Geometry: final body of the model. Coordinates: model frame, mm. A direction names the side the tool comes from. Coordinates: 2 decimals unless noted, no trailing zeros. Order: outer loops, then holes, each group sorted by start corner. A loop starts at its lowest first (then second) coordinate and runs counter-clockwise, first axis right, second up. Notation, with made-up numbers: (35, 67) -> (91, 67) arc R21 ccw to (91, 81) -> close; hole circle Ø2 at (-2, 12.25). An arc over 180 degrees is marked (long way). Use one line per item in the form item = value.
```python
from build123d import *

# Parameters (mm, degrees)
SKETCH1_R           = 1.475
SKETCH1_R_2         = 22.5
SKETCH1_R_3         = 11
SKETCH1_W           = 24.7
SKETCH1_H           = 4.85
BOSS_EXTRUDE1_DEPTH = 5


with BuildPart() as part:
    # Sketch1 → Boss-Extrude1 (new body)
    with BuildSketch(Plane.XY):
        with BuildLine():
            Line((-139.300035894, 89.802561211), (-24.748737342, -24.748737342))
            ThreePointArc((-24.748737342, -24.748737342), (24.748737342, -24.748737342), (24.748737342, 24.748737342))
            Line((24.748737342, 24.748737342), (-54.672802234, 104.170276917))
            Line((-54.672802234, 104.170276917), (-76.622366364, 126.119841047))
            ThreePointArc((-76.622366364, 126.119841047), (-78.790093877, 129.364074535), (-79.551298552, 133.190908859))
            Line((-79.551298552, 133.190908859), (-79.551298552, 164.551298552))
            Line((-79.551298552, 164.551298552), (-89.351298552, 164.551298552))
            Line((-89.351298552, 164.551298552), (-89.351298552, 169.551298552))
            Line((-89.351298552, 169.551298552), (-96.351298552, 169.551298552))
            Line((-96.351298552, 169.551298552), (-96.351298552, 174.551298552))
            Line((-96.351298552, 174.551298552), (-109.751298552, 174.551298552))
            Line((-109.751298552, 174.551298552), (-109.751298552, 169.551298552))
            Line((-109.751298552, 169.551298552), (-119.351298552, 169.551298552))
            Line((-119.351298552, 169.551298552), (-119.351298552, 174.551298552))
            Line((-119.351298552, 174.551298552), (-132.751298552, 174.551298552))
            Line((-132.751298552, 174.551298552), (-132.751298552, 169.551298552))
            Line((-132.751298552, 169.551298552), (-139.751298552, 169.551298552))
            Line((-139.751298552, 169.551298552), (-139.751298552, 164.551298552))
            Line((-139.751298552, 164.551298552), (-149.551298552, 164.551298552))
            Line((-149.551298552, 164.551298552), (-149.551298552, 114.551298552))
            ThreePointArc((-149.551298552, 114.551298552), (-146.88708219, 101.157378419), (-139.300035894, 89.802561211))
        make_face()
        with BuildLine():
            Line((-78.771695424, 51.335952314), (-89.378297142, 61.942554032))
            ThreePointArc((-89.378297142, 61.942554032), (-89.378297142, 65.336666582), (-85.984184592, 65.336666582))
            Line((-85.984184592, 65.336666582), (-75.377582874, 54.730064864))
            ThreePointArc((-75.377582874, 54.730064864), (-75.377582874, 51.335952314), (-78.771695424, 51.335952314))
        make_face(mode=Mode.SUBTRACT)
        with BuildLine():
            ThreePointArc((-68.165093707, 64.770981156), (-68.165093707, 68.165093706), (-64.770981157, 68.165093706))
            Line((-64.770981157, 68.165093706), (-54.164379439, 57.558491989))
            ThreePointArc((-54.164379439, 57.558491989), (-54.164379439, 54.164379439), (-57.558491988, 54.164379439))
            Line((-57.558491988, 54.164379439), (-68.165093707, 64.770981156))
        make_face(mode=Mode.SUBTRACT)
        with Locations((-20.506096654, -20.506096654)):
            Circle(SKETCH1_R, mode=Mode.SUBTRACT)
        with Locations((-56.568542495, 14.142135624)):
            Circle(SKETCH1_R, mode=Mode.SUBTRACT)
        with Locations((20.506096654, -20.506096654)):
            Circle(SKETCH1_R, mode=Mode.SUBTRACT)
        Circle(SKETCH1_R_2, mode=Mode.SUBTRACT)
        with Locations((-55.401816306, 29.450997436)):
            Circle(SKETCH1_R, mode=Mode.SUBTRACT)
        with BuildLine():
            ThreePointArc((-47.623641713, 19.5515025), (-47.623641713, 21.672822843), (-45.502321369, 21.672822843))
            Line((-45.502321369, 21.672822843), (-41.966787463, 18.137288937))
            ThreePointArc((-41.966787463, 18.137288937), (-41.966787463, 16.015968594), (-44.088107807, 16.015968594))
            Line((-44.088107807, 16.015968594), (-47.623641713, 19.5515025))
        make_face(mode=Mode.SUBTRACT)
        with BuildLine():
            ThreePointArc((-47.72970773, 37.123106012), (-47.72970773, 40.658639918), (-44.194173824, 40.658639918))
            Line((-44.194173824, 40.658639918), (-30.0520382, 26.516504294))
            ThreePointArc((-30.0520382, 26.516504294), (-30.0520382, 22.980970389), (-33.587572106, 22.980970389))
            Line((-33.587572106, 22.980970389), (-47.72970773, 37.123106012))
        make_face(mode=Mode.SUBTRACT)
        with Locations((-20.506096654, 20.506096654)):
            Circle(SKETCH1_R, mode=Mode.SUBTRACT)
        with BuildLine():
            ThreePointArc((-40.658639918, 44.194173824), (-40.658639918, 47.72970773), (-37.123106012, 47.72970773))
            Line((-37.123106012, 47.72970773), (-22.980970389, 33.587572106))
            ThreePointArc((-22.980970389, 33.587572106), (-22.980970389, 30.0520382), (-26.516504294, 30.0520382))
            Line((-26.516504294, 30.0520382), (-40.658639918, 44.194173824))
        make_face(mode=Mode.SUBTRACT)
        with BuildLine():
            ThreePointArc((-35.001785669, 49.851028074), (-35.001785669, 53.38656198), (-31.466251763, 53.38656198))
            Line((-31.466251763, 53.38656198), (-17.324116139, 39.244426356))
            ThreePointArc((-17.324116139, 39.244426356), (-17.324116139, 35.70889245), (-20.859650045, 35.70889245))
            Line((-20.859650045, 35.70889245), (-35.001785669, 49.851028074))
        make_face(mode=Mode.SUBTRACT)
        with BuildLine():
            ThreePointArc((-29.344931419, 55.507882323), (-29.344931419, 59.043416229), (-25.809397513, 59.043416229))
            Line((-25.809397513, 59.043416229), (-11.66726189, 44.901280605))
            ThreePointArc((-11.66726189, 44.901280605), (-11.66726189, 41.365746699), (-15.202795796, 41.365746699))
            Line((-15.202795796, 41.365746699), (-29.344931419, 55.507882323))
        make_face(mode=Mode.SUBTRACT)
        with Locations((-14.142135624, 56.568542495)):
            Circle(SKETCH1_R, mode=Mode.SUBTRACT)
        with Locations((20.506096654, 20.506096654)):
            Circle(SKETCH1_R, mode=Mode.SUBTRACT)
        with Locations((-114.551298552, 84.551298552)):
            Circle(SKETCH1_R, mode=Mode.SUBTRACT)
        with Locations((-130.051298552, 99.051298552)):
            Circle(SKETCH1_R, mode=Mode.SUBTRACT)
        with Locations((-114.551298552, 114.551298552)):
            Circle(SKETCH1_R_3, mode=Mode.SUBTRACT)
        with BuildLine():
            ThreePointArc((-86.549870017, 83.155757468), (-86.549870017, 86.549870017), (-83.155757468, 86.549870017))
            Line((-83.155757468, 86.549870017), (-72.54915575, 75.943268299))
            ThreePointArc((-72.54915575, 75.943268299), (-72.54915575, 72.54915575), (-75.943268299, 72.54915575))
            Line((-75.943268299, 72.54915575), (-86.549870017, 83.155757468))
        make_face(mode=Mode.SUBTRACT)
        with BuildLine():
            ThreePointArc((-65.336666582, 85.984184592), (-65.336666582, 89.378297142), (-61.942554032, 89.378297142))
            Line((-61.942554032, 89.378297142), (-51.335952314, 78.771695424))
            ThreePointArc((-51.335952314, 78.771695424), (-51.335952314, 75.377582874), (-54.730064864, 75.377582874))
            Line((-54.730064864, 75.377582874), (-65.336666582, 85.984184592))
        make_face(mode=Mode.SUBTRACT)
        with Locations((-99.051298552, 99.051298552)):
            Circle(SKETCH1_R, mode=Mode.SUBTRACT)
        with Locations((-64.396887007, 105.308740477)):
            Circle(SKETCH1_R, mode=Mode.SUBTRACT)
        with Locations((-130.051298552, 130.051298552)):
            Circle(SKETCH1_R, mode=Mode.SUBTRACT)
        with Locations((-136.551298552, 152.551298552)):
            Circle(SKETCH1_R, mode=Mode.SUBTRACT)
        with Locations((-114.551298552, 162.126298552)):
            Rectangle(SKETCH1_W, SKETCH1_H, mode=Mode.SUBTRACT)
        with Locations((-99.051298552, 130.051298552)):
            Circle(SKETCH1_R, mode=Mode.SUBTRACT)
        with Locations((-92.551298552, 152.551298552)):
            Circle(SKETCH1_R, mode=Mode.SUBTRACT)
    extrude(amount=-BOSS_EXTRUDE1_DEPTH)


solid = part.part
```
1) Section D-D, the plane z = -3.65. Give the number of separate pieces and of enclosed holes in the cut face, and give its area (3 significant figures).
Results found:
separate_pieces = 1
enclosed_holes = 27
area = 14,100 mm2
2) Access query for faces 1 (the flat face through (-62.788, 59.393, -2.465)), 2 (the flat face through (-93, 169.551, -2)), 3 (the flat face through (-119.351, 172, -2)), 4 (the flat face through (-136, 169.551, -2)). Directions: +Z, -Z, +X, -X, +Y, -Y. A direction counts if a zero-diameter tool reaches every point of the face in a straight line with its end or side. Return the directions, or none.
Results found:
face_1 = +Z, -Z
face_2 = +Z, -Z, +X, +Y
face_3 = +Z, -Z, +Y
face_4 = +Z, -Z, -X, +Y
3) Pull-direction query (Y, two-part tool) for faces 5 (the cylindrical face through (-146.96, 101.34, -2.46)), 6 (the flat face through (-79.551, 149, -2)), 7 (the cylindrical face through (-22.943, 30.091, -2.465)), 8 (the flat face through (-77.927, 81.321, -2.465)); classes: released by +Y, released by -Y, zero draft, split by the parting line, or undercut.
Results found:
face_5 = released by -Y
face_6 = zero draft
face_7 = undercut
face_8 = undercut
4) Contact query for flat-ended pins moving along their axis: P1, Ø2.5, axis at y = 173, z = -1.5, coming from the -X side; P2, Ø1, axis at x = -76.5, z = -3.5, coming from the -Y side; P3, Ø2.5, axis at y = 171, z = -1.5, coming from the +X side. Output: stop coordinate, or through.
Results found:
P1 = -132.75
P2 = 26.5
P3 = -96.35
5) Section A-A, the plane y = -4. Output: boundary loops of the cut face in (x, z).
Results found:
outline = (-45.5, -5) -> (-22.14, -5) -> (-22.14, 0) -> (-45.5, 0) -> close; (22.14, -5) -> (34.77, -5) -> (34.77, 0) -> (22.14, 0) -> close
6) Section B-B, the plane x = 0. Output: boundary loops of the cut face in (y, z).
Results found:
outline = (-35, -5) -> (-22.5, -5) -> (-22.5, 0) -> (-35, 0) -> close; (22.5, -5) -> (49.5, -5) -> (49.5, 0) -> (22.5, 0) -> close
7) Material intervals for probe 1 along Y at (x, z) = (-81.5, -0.65); probe 2 along Y at (x, z) = (-122, -0.25); probe 3 along X at (y, z) = (39, -1.6), sorted ascending. Write a range as from..to.
Results found:
probe_1 = 32..54.06, 60.85..78.11, 84.89..164.55
probe_2 = 72.5..106.46, 122.65..159.7, 164.55..174.55
probe_3 = -88.5..-48.46, -42.54..-35.46, -28.39..-24.15, -17.11..10.5
8) Section C-C, the plane y = 146. Output: boundary loops of the cut face in (x, z).
Results found:
outline = (-149.55, -5) -> (-79.55, -5) -> (-79.55, 0) -> (-149.55, 0) -> close
